from build123d import *

# Parameters (mm, degrees)
F0_R     = 50.211231
F1_DEPTH = 500
F2_R     = 5.08
F3_R     = 5.08


with BuildPart() as f1:
    # F0 (on Top) → F1 (new body, symmetric)
    with BuildSketch(Plane.XY):
        Circle(F0_R)
    extrude(amount=F1_DEPTH, both=True)

    # F2
    f2_edges = [f1.edges().sort_by_distance(p)[0] for p in [
        (-50.211231, 0, -500),
    ]]
    fillet(f2_edges, radius=F2_R)

    # F3
    f3_edges = [f1.edges().sort_by_distance(p)[0] for p in [
        (-50.211231, 0, 500),
    ]]
    fillet(f3_edges, radius=F3_R)


solid = f1.part
Here's how the part is built. I have some questions about the finished solid (model axes, mm). Coordinates: 2 decimals unless noted, no trailing zeros. Order: outer loops, then holes, each group sorted by start corner. A loop starts at its lowest first (then second) coordinate and runs counter-clockwise, first axis right, second up.
Item 1: For P1, Ø1, axis at x = 40, z = -226, coming from the -Y side; P2, Ø1.5, axis at y = 18.5, z = -253.5, coming from the +X side; P3, Ø2, axis at x = 30.5, y = -37.5, coming from the -Z side, each with a flat end and sliding along its axis, tell me the tip position at first contact or that it passes through.
Result sheet:
P1: stops at y = -31
P2: stops at x = 46.97
P3: stops at z = -499.5
Item 2: I need wall thicknesses on line 1 (Y direction, x = 3, z = -213.5); line 2 (Z direction, x = -5.5, y = 46). Which ranges of each line are inside material? Lowest first, please.
Result sheet:
line 1: y = -50.12 to 50.12
line 2: z = -499.86 to 499.86
Item 3: If we section it at A-A on z = -353.5: List the corners of the cut face in (x, y) for me.
Result sheet:
outline: circle Ø100.42 at (0, 0)
